Geometry: final body of the model. Coordinates: model frame, mm. Round coordinates to 2 decimals unless told otherwise and drop trailing zeros. Loops run counter-clockwise (first coordinate to the right, second up) from the corner with the lowest first, then second, coordinate; pieces in that order, holes last. Notation, with made-up numbers: M 69,-6.5 L 119,-6.5 A8 cw 119,-0.5 Z; hole C -18.75,-15 d7. An arc over 180 degrees is marked long. Return JSON: item names as keys, results as strings.
from build123d import *

# Parameters (mm, degrees)
F0_R     = 2.5
F1_DEPTH = 6
F2_R     = 3


with BuildPart() as f1:
    # F0 (on Front) → F1 (new body)
    with BuildSketch(Plane.XZ):
        with BuildLine():
            Line((0, 9), (0, 0))
            Line((0, 0), (9, 0))
            ThreePointArc((9, 0), (2.6360389693, 2.6360389693), (0, 9))
        make_face()
        with BuildLine():
            ThreePointArc((0, 9), (2.6360389693, 2.6360389693), (9, 0))
            ThreePointArc((9, 0), (15.3639610307, 2.6360389693), (18, 9))
            ThreePointArc((18, 9), (15.3639610307, 15.3639610307), (9, 18))
            ThreePointArc((9, 18), (2.6360389693, 15.3639610307), (0, 9))
        make_face()
        with Locations((9, 9)):
            Circle(F0_R, mode=Mode.SUBTRACT)
        with BuildLine():
            Line((0, 18), (0, 9))
            ThreePointArc((0, 9), (2.6360389693, 15.3639610307), (9, 18))
            Line((9, 18), (0, 18))
        make_face()
    extrude(amount=F1_DEPTH)

    # F2
    f2_edges = [f1.edges().sort_by_distance(p)[0] for p in [
        (0, -3, 18),
        (0, -3, 0),
    ]]
    fillet(f2_edges, radius=F2_R)


solid = f1.part
Q1. Section query B-B (y = -2.95). Output: boundary loops of the cut face in (x, z).
Determined:
{"outline": "M 0,3 A3 ccw 3,0 L 9,0 A9 ccw 9,18 L 3,18 A3 ccw 0,15 Z; hole C 9,9 d5"}
Q2. Material intervals for L1, parallel to Z at x = 9, y = -3.4; L2, parallel to X at y = -5.05, z = 10.75; L3, parallel to Z at x = 7.25, y = -4.4, sorted ascending.
Determined:
{"L1": "z = 0 to 6.5, 11.5 to 18", "L2": "x = 0 to 7.21, 10.79 to 17.83", "L3": "z = 0 to 7.21, 10.79 to 18"}
Q3. Section query D-D (x = 14). Output: boundary loops of the cut face in (y, z).
Determined:
{"outline": "M -6,1.52 L 0,1.52 L 0,16.48 L -6,16.48 Z"}
Q4. Section query A-A (x = 8.75). Output: boundary loops of the cut face in (y, z), plus the area to 3 significant figures.
Determined:
{"outline": "M -6,0 L 0,0 L 0,6.51 L -6,6.51 Z; M -6,11.49 L 0,11.49 L 0,18 L -6,18 Z", "area": "78.2 mm^2"}
Q5. Pull-direction query (Z, two-part tool) for faces 1 (the flat face through (7, -6, 7)), 2 (the flat face through (6, -3, 18)), 3 (the cylindrical face through (8.46, -2.96, 6.56)); classes: pulls with the +Z half, pulls with the -Z half, needs draft (parallel to the pull), parting line crosses it, or undercut.
Determined:
{"face 1": "needs draft", "face 2": "pulls with the +Z half", "face 3": "undercut"}
Q6. Section query C-C (z = 6.75). Output: boundary loops of the cut face in (x, y), plus the area to 3 significant figures.
Determined:
{"outline": "M 0,-6 L 7.91,-6 L 7.91,0 L 0,0 Z; M 10.09,-6 L 17.71,-6 L 17.71,0 L 10.09,0 Z", "area": "93.2 mm^2"}
Q7. Pin query (flat end, axial travel): pin 1 (3 mm diameter, centred on x = 11, y = -4, fed in from +Z); pin 2 (2 mm diameter, centred on x = 12, y = -3, fed in from -Z); pin 3 (8 mm diameter, centred on x = 9, z = 9, fed in from -Y). Return the tip coordinate at first contact, or that it passes through.
Determined:
{"pin 1": "stops at z = 17.99", "pin 2": "stops at z = 0.23", "pin 3": "stops at y = -6"}
